Can you work these out from the model? Positions are in its coordinate system, mm. Give positions to 0.01 mm unless a question says otherwise; leave off trailing zeros. Loops run counter-clockwise (first coordinate to the right, second up) from the corner with the lowest first, then second, coordinate; pieces in that order, holes last. Notation, with made-up numbers: M 45.25,78 L 72.25,78 A17 cw 72.25,85 Z; hole C 36,-36.75 d4. An arc over 180 degrees is marked long. Answer as a JSON object with one key per item and string values.
```python
from build123d import *

# Parameters (mm, degrees)
F0_R     = 23
F0_R_2   = 20
F1_DEPTH = 20
F2_R     = 23
F3_DEPTH = 3
F4_R     = 1


with BuildPart() as f1:
    # F0 (on Top) → F1 (new body)
    with BuildSketch(Plane.XY):
        Circle(F0_R)
        Circle(F0_R_2, mode=Mode.SUBTRACT)
    extrude(amount=F1_DEPTH)

    # F2 (on Top) → F3 (join)
    with BuildSketch(Plane.XY):
        Circle(F2_R)
    extrude(amount=F3_DEPTH)

    # F4
    f4_edges = [f1.edges().sort_by_distance(p)[0] for p in [
        (-20, 0, 20),
        (-23, 0, 20),
        (-23, 0, 0),
    ]]
    fillet(f4_edges, radius=F4_R)


solid = f1.part
```
1) Suppose I cut it at B-B, the plane z = 4. Write out the boundary of the cut face in (x, y), and give its area (3 significant figures).
Answer list:
{"outline": "C 0,0 d46; hole C 0,0 d40", "area": "405 mm^2"}
2) Will these pins go through, and if not, where does the flat tip stop? pin 1 Ø2 at (x, z) = (1.5, 10.5) entering from +Y; pin 2 Ø8 at (x, y) = (7.5, -17) entering from +Z; pin 3 Ø1.5 at (x, z) = (9.5, 12) entering from -Y; pin 4 Ø2 at (x, y) = (8, 5) entering from +Z.
Answer list:
{"pin 1": "y = 22.99", "pin 2": "z = 20", "pin 3": "y = -21.27", "pin 4": "z = 3"}
3) Suppose I cut it at A-A, the plane y = 0. Write out the boundary of the cut face in (x, z).
Answer list:
{"outline": "M -23,1 A1 ccw -22,0 L 22,0 A1 ccw 23,1 L 23,19 A1 ccw 22,20 L 21,20 A1 ccw 20,19 L 20,3 L -20,3 L -20,19 A1 ccw -21,20 L -22,20 A1 ccw -23,19 Z"}
4) If we mould it in two halves opening along Y, with no side actions, what happens to faces 1 (the cylindrical face through (-4.336, -19.524, 10.888)), 2 (the flat face through (0, 0, 0)), 3 (the cylindrical face through (-2.994, 22.804, 9.874))? For each: +Y half, -Y half, draft (parallel to the pull), parting line (faces both ways), or undercut.
Answer list:
{"face 1": "undercut", "face 2": "draft", "face 3": "parting line"}
5) Please list where these lines run through material, in increasing order: line 1 along Y through (x, z) = (0, 8.75); line 2 along Z through (x, y) = (-1.5, -2); line 3 along X through (y, z) = (-14, 12.5). Write a range as from..to.
Answer list:
{"line 1": "-23..-20, 20..23", "line 2": "0..3", "line 3": "-18.25..-14.28, 14.28..18.25"}
